Can you work these out from the drawing? Everything is in mm from the part's minimum corner. A direction names the side the tool comes from. Round coordinates to 2 decimals unless told otherwise and drop trailing zeros. Loops run counter-clockwise (first coordinate to the right, second up) from the corner with the lowest first, then second, coordinate; pieces in that order, holes last. Notation, with made-up numbers: M 8.25,-38.5 L 49.25,-38.5 A25 ccw 49.25,-6.5 Z; hole C -14.75,59 d8. An arc over 180 degrees is marked long. One line per question, with ' | ' between items. Start each with the question number.
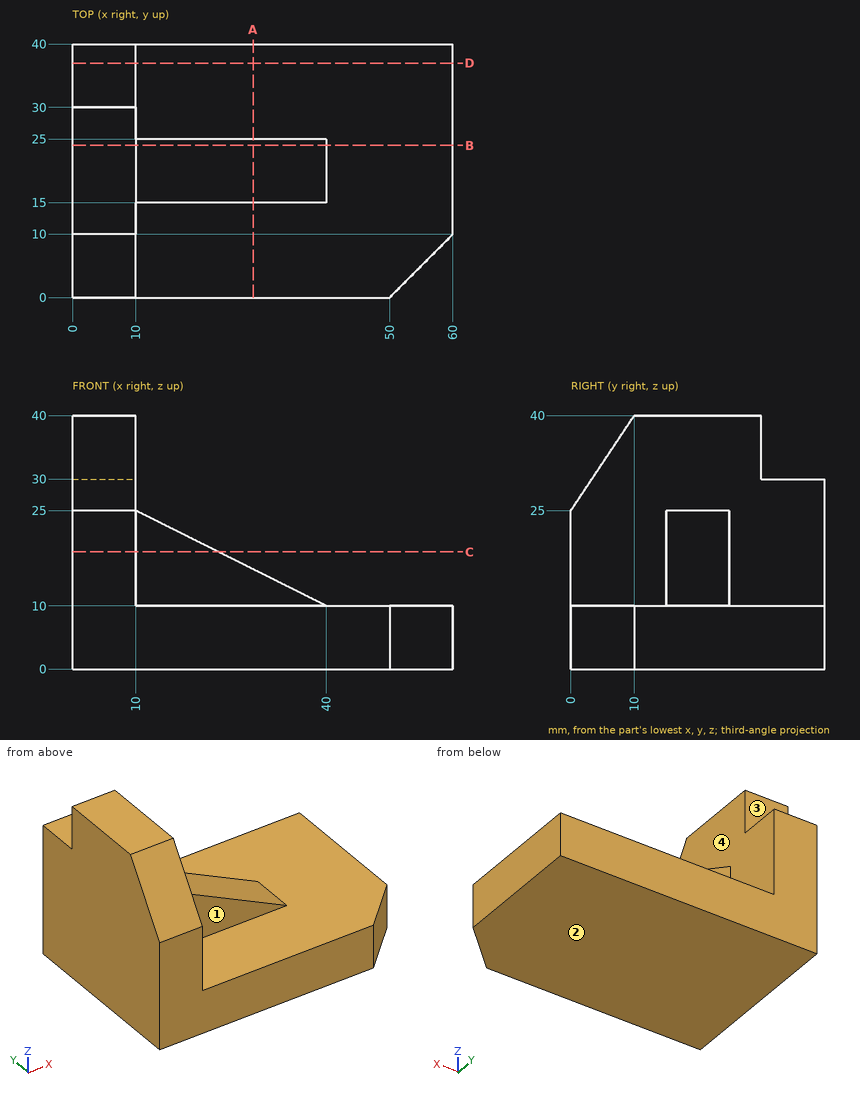
1) Imagine slicing it at C-C (z = 18.5). Write out the boundary of the cut face in (x, y), then the cut area to 3 significant figures.
2) Imagine slicing it at A-A (x = 28.5). Write out the boundary of the cut face in (y, z), then the cut area to 4 significant figures.
3) Imagine slicing it at D-D (y = 37). Write out the boundary of the cut face in (x, z).
4) For the marked faces 1, 2, 3 and 4, which set-ups out of +Z, -Z, +X, -X, +Y, -Y let a thin tool reach every point of the face, with its end or its side?
5) Imagine slicing it at B-B (y = 24). Write out the boundary of the cut face in (x, z), then the cut area to 4 significant figures.
6) I'm going to push flat-ended pins straight in: pin 1 Ø7.5 at (x, z) = (25, 19.5) entering from -Y; pin 2 Ø5 at (y, z) = (4.5, 19) entering from +X; pin 3 Ø20 at (x, y) = (25.5, 14.5) entering from +Z. Where does each tip first touch, or does it pass through?
7) Please list where these lines run through material, in increasing order: L1, parallel to X at y = 7, z = 25; L2, parallel to X at y = 21, z = 15. Write a range as from..to.
Results are:
1) outline: M 0,0 L 10,0 L 10,15 L 23,15 L 23,25 L 10,25 L 10,40 L 0,40 Z | area: 530 mm²
2) outline: M 0,0 L 40,0 L 40,10 L 25,10 L 25,15.75 L 15,15.75 L 15,10 L 0,10 Z | area: 457.5 mm²
3) outline: M 0,0 L 60,0 L 60,10 L 10,10 L 10,30 L 0,30 Z
4) face 1: +Z, +X, -Y | face 2: -Z, +X, -X, +Y, -Y | face 3: +Z, +X, -X, +Y | face 4: +Z, +X
5) outline: M 0,0 L 60,0 L 60,10 L 40,10 L 10,25 L 10,40 L 0,40 Z | area: 1,125 mm²
6) pin 1: y = 15 | pin 2: x = 10 | pin 3: z = 22.24
7) L1: 0..10 | L2: 0..30
